Check sheet for the modelled part. Datum: model origin and axes. Units: mm. A direction names the side the tool comes from. Round coordinates to 2 decimals unless told otherwise and drop trailing zeros. Write each loop counter-clockwise with the first axis right and the second up, starting at its lowest first coordinate (ties: lowest second). Pieces come first, ordered by that corner, then holes.
Item 1: Section check B-B, the plane y = 2. State how many separate pieces and enclosed holes the cut face has, plus the area to 3 significant figures.
Item 2: Set-up check for faces 4 (the flat face through (14.75, -2, 34)), 5 (the flat face through (-10.485, -2, 0)), 6 (the flat face through (12.185, 3.2, 0.1)): record each of +Z, -Z, +X, -X, +Y, -Y from which the full face is reachable in a straight line by a thin tool's end or side.
Item 3: Material ranges on line 1 along Y through (x, z) = (0, -20); line 2 along X through (y, z) = (0.25, -7); line 3 along Y through (x, z) = (0, 35.5), recorded low to high.
Item 4: Section check C-C, the plane z = 35.5. Record the cut outline in (x, y), plus the area to 3 significant figures.
Item 5: Section check A-A, the plane z = -3. Record the cut outline in (x, y) (3 decimals).
Item 6: Depth check by flat-ended pin: pin 1 (5 mm diameter, centred on y = -1, z = -34, fed in from -X); pin 2 (1 mm diameter, centred on y = -0.5, z = -12.5, fed in from +X); pin 3 (3.5 mm diameter, centred on y = -2.5, z = -35, fed in from +X). Enter the tip coordinate at first touch or a pass-through.
Item 7: Release check for a two-part mould opening along Y. For faces 1 (the flat face through (9.7, -3, 49.2)), 2 (the flat face through (11, 0, 0)), 3 (the cylindrical face through (0, 1, 20)) record: pulls with the +Y half, pulls with the -Y half, needs draft (parallel to the pull), parting line crosses it, or undercut.
Autodesk Inventor part; units mm, degrees
ref_plane "YZ Plane" through (0, 0, 0) normal (1, 0, 0) x (0, 1, 0)
ref_plane "XZ Plane" through (0, 0, 0) normal (0, 1, 0) x (-1, 0, 0)
ref_plane "XY Plane" through (0, 0, 0) normal (0, 0, 1) x (1, 0, 0)
sketch "Chamber_outline" plane through (0, 0, 0) normal (0, 1, 0) x (-1, 0, 0)
  line L0 (0, -6.495) -> (0, 6.495) construction
  line L1 (12.185, -6.495) -> (12.185, 6.495)
  line L2 (-12.185, 6.495) -> (-12.185, -6.495)
  arc A0 (-12.185, -6.495) -> (12.185, -6.495) centre (0, -6.495) ccw
  arc A1 (12.185, 6.495) -> (-12.185, 6.495) centre (0, 6.495) ccw
  line L3 (15.7049, -6.495) -> (15.7049, 6.495)
  arc A2 (15.7049, 6.495) -> (-15.7049, 6.495) centre (0, 6.495) ccw
  line L4 (-15.7049, 6.495) -> (-15.7049, -6.495)
  arc A3 (-15.7049, -6.495) -> (15.7049, -6.495) centre (0, -6.495) ccw
  line L5 (12.185, 0) -> (-12.185, 0)
  line L6 (14.7497, -11.8886) -> (14.7497, -56.8886)
  line L7 (14.7497, -56.8886) -> (-14.7497, -56.8886)
  line L8 (-14.7497, -56.8886) -> (-14.7497, -11.8886)
  line L9 (14.7497, 11.8886) -> (14.7497, 56.8886)
  line L10 (14.7497, 56.8886) -> (-14.7497, 56.8886)
  line L11 (-14.7497, 56.8886) -> (-14.7497, 11.8886)
  line L12 (10.485, -6.495) -> (10.485, 6.495)
  arc A4 (10.485, 6.495) -> (-10.485, 6.495) centre (0, 6.495) ccw
  line L13 (-10.485, 6.495) -> (-10.485, -6.495)
  arc A5 (-10.485, -6.495) -> (10.485, -6.495) centre (0, -6.495) ccw
  point P0 (0, 0)
  point P1 (0, 0)
  point P2 (0, 0)
  point P3 (0, -56.8886)
  point P4 (0, 56.8886)
  point P5 (-14.7497, 11.8886)
  point P6 (14.7497, 11.8886)
  point P7 (0, -18.68)
  point P8 (0, 18.68)
  dimension "d18" = 24.37
  dimension "d26" = 1.7
  dimension "d58" = 45
  dimension "d82" = 37.36
extrude "Extrusion3" add sketch "Chamber_outline" along normal blind 4.5 contours A3 L4 A2 L3
extrude "Extrusion4" add sketch "Chamber_outline" along normal blind 0.5 contours L6 L7 L8 A3 | A2 L11 L10 L9
extrude "Extrusion5" add sketch "Chamber_outline" against normal blind 4 contours A0 L2 L5 L13 A5 L12 L1 | L5 L12 A4 L13 L2 A1 L1 | A3 L4 A2 L3 | L6 L7 L8 A3 | A2 L11 L10 L9
fillet "Fillet1" radius 10 2 edges at (-14.7497, -2, 11.8886) (-14.7497, 0.25, 11.8886)
fillet "Fillet2" radius 10 6 edges at (-14.7497, -2, -11.8886) (-14.7497, 0.25, -11.8886) (14.7497, 0.25, -11.8886) (14.7497, -2, -11.8886) (14.7497, 0.25, 11.8886) (14.7497, -2, 11.8886)
fillet "Fillet3" radius 2 8 edges at (-14.7497, -2, -56.8886) (-14.7497, 0.25, -56.8886) (-14.7497, -2, 56.8886) (-14.7497, 0.25, 56.8886) (14.7497, -2, 56.8886) (14.7497, 0.25, 56.8886) (14.7497, -2, -56.8886) (14.7497, 0.25, -56.8886)
sketch "Sketch9" plane through (0, -4, 0) normal (0, -1, 0) x (1, 0, 0)
  line L0 (0.801, 42.3276) -> (0.801, 45.3727) construction
  line L1 (0.801, 45.3727) -> (3.851, 45.3727) construction
  line L2 (3.851, 45.3727) -> (3.851, 42.3276) construction
  line L3 (3.851, 42.3276) -> (0.801, 42.3276) construction
  line L4 (10.801, 43.349) -> (0.801, 43.349)
  line L5 (0.801, 43.349) -> (0.801, 47.602)
  spline S0 degree 2 poles (0.801, 47.602) (0.801, 49.2102) (1.3422, 50.6584) (2.7141, 51.5349) (3.6059, 51.5349) knots 0 0 0 1 2 3 3 3
  spline S1 degree 2 poles (3.6059, 51.5349) (4.7263, 51.5349) (6.1973, 50.2163) (6.3879, 48.8977) knots 0 0 0 1 2 2 2
  spline S2 degree 2 poles (6.3879, 48.8977) (6.769, 49.5532) (7.6836, 50.4069) (8.8498, 51.131) knots 0 0 0 1 2 2 2
  line L6 (8.8498, 51.131) -> (10.801, 52.3505)
  line L7 (10.801, 52.3505) -> (10.801, 49.9343)
  line L8 (10.801, 49.9343) -> (8.6211, 48.4785)
  spline S3 degree 2 poles (8.6211, 48.4785) (7.455, 47.6935) (6.8452, 47.1218) (6.6242, 46.4816) (6.6242, 45.7804) knots 0 0 0 1 2 3 3 3
  line L9 (6.6242, 45.7804) -> (6.6242, 45.3688)
  line L10 (6.6242, 45.3688) -> (10.801, 45.3688)
  line L11 (10.801, 45.3688) -> (10.801, 43.349)
  line L12 (5.0312, 45.3688) -> (5.0312, 46.8627)
  spline S4 degree 2 poles (5.0312, 46.8627) (5.0312, 48.3185) (4.7873, 49.0426) (4.1851, 49.4541) (3.7355, 49.4541) knots 0 0 0 1 2 3 3 3
  spline S5 degree 2 poles (3.7355, 49.4541) (3.2324, 49.4541) (2.6074, 48.913) (2.5236, 48.4252) knots 0 0 0 1 2 2 2
  spline S6 degree 2 poles (2.5236, 48.4252) (2.4931, 48.1737) (2.4931, 46.9465) knots 0 0 0 1 1 1
  line L13 (2.4931, 46.9465) -> (2.4931, 45.3688)
  line L14 (2.4931, 45.3688) -> (5.0312, 45.3688)
  point P0 (0, 0)
extrude "Extrusion14" cut sketch "Sketch9" against normal blind 2
sketch "Sketch3" plane through (15.7049, 4.5, 6.495) normal (1, 0, 0) x (0, 0, -1)
  circle A0 centre (6.5, -2.5) radius 1
  line L0 (0, 0) -> (12.99, 0)
  circle A1 centre (14.5, -2.5) radius 1
  circle A2 centre (-1.5, -2.5) radius 1
  point P0 (6.495, -4.5)
  dimension "d41" = 2
  dimension "d43" = 2.5
  dimension "d85" = 2
  dimension "d86" = 2
  dimension "d87" = 8
  dimension "d88" = 8
extrude "Extrusion6" cut sketch "Sketch3" against normal through all
sketch "Sketch4" plane through (-12.7497, 0.5, 56.8886) normal (0, 0, 1) x (1, 0, 0)
  circle A0 centre (12.7497, 1.5) radius 1
  line L0 (28.4546, 4) -> (-2.9552, 4)
  point P0 (12.7497, -0.5)
  point P1 (12.7497, 4)
  dimension "d36" = 2
  dimension "d42" = 2.5
extrude "Extrusion7" cut sketch "Sketch4" against normal through all
sketch "Sketch5" plane through (0, -4, 0) normal (0, -1, 0) x (1, 0, 0)
  line L0 (-10.485, -6.495) -> (-10.485, 6.495)
  line L1 (-10.485, -6.495) -> (-8.4271, -6.495)
  line L2 (-7.9121, 0.245) -> (-7.9121, 6.495)
  line L3 (-7.9121, 6.495) -> (-10.485, 6.495)
  line L4 (10.485, -6.495) -> (10.485, 6.495)
  line L5 (10.485, -6.495) -> (8.4271, -6.495)
  line L6 (8.3305, -0.2609) -> (8.3305, 6.495)
  line L7 (8.3305, 6.495) -> (10.485, 6.495)
  arc A0 (10.485, 6.495) -> (-10.485, 6.495) centre (0, 6.495) ccw
  arc A1 (-10.485, -6.495) -> (10.485, -6.495) centre (0, -6.495) ccw
  arc A2 (-10.485, -6.495) -> (10.485, -6.495) centre (0, -6.495) ccw
  line L8 (-7.079, -14.2295) -> (-5.3711, -11.1831)
  line L9 (-5.3711, -11.1831) -> (-3.3516, -12.3154)
  line L10 (-3.3516, -12.3154) -> (-5.1945, -15.6028)
  line L11 (-7.4267, 14.3644) -> (-5.7188, 11.3181)
  line L12 (-5.7188, 11.3181) -> (-3.6001, 12.5059)
  line L13 (-3.6001, 12.5059) -> (-5.4497, 15.8051)
  line L14 (3.586, 12.9764) -> (5.1976, 15.6011)
  line L15 (5.8011, 11.7346) -> (3.586, 12.9764)
  line L16 (7.1611, 14.1536) -> (5.8011, 11.7346)
  line L17 (-10.485, -6.495) -> (10.8395, -6.495)
  line L18 (1.9666, 16.7939) -> (1.9666, -0.2609)
  line L19 (-2.0003, -16.7874) -> (-2.0003, -6.495)
  line L20 (-1.0812, 0.245) -> (-1.0812, 16.9241)
  line L21 (4.8643, -15.7834) -> (4.8643, -6.495)
  line L22 (-7.9121, 0.245) -> (-1.0812, 0.245)
  line L23 (1.9666, -0.2609) -> (8.3305, -0.2609)
  point P0 (0, 0)
  point P1 (1.5355, -6.495)
  point P2 (-7.079, -14.2295)
  point P3 (-5.1945, -15.6028)
  point P4 (-5.3016, 15.5409)
  point P5 (-7.2574, 14.0624)
  point P6 (7.5128, 14.2848)
  point P7 (5.4529, 15.8033)
  point P8 (8.4271, -6.495)
  point P9 (4.8643, -15.7834)
sketch "Sketch6" plane through (0, -4, 0) normal (0, -1, 0) x (1, 0, 0)
  ellipse E0 centre (0, -5) end of major axis (0.355, -4.9802) minor radius 0.3556
  circle A0 centre (1, -5.9999) radius 0.3556
  circle A1 centre (0, -5.9999) radius 0.3556
  circle A2 centre (-1, -6) radius 0.3556
  circle A3 centre (-1, -4.9999) radius 0.3556
  circle A4 centre (1, -5) radius 0.3556
  circle A5 centre (1, -6.9999) radius 0.3556
  ellipse E1 centre (0, -7) end of major axis (0.3551, -6.9801) minor radius 0.3556
  ellipse E2 centre (-1, -7) end of major axis (-0.645, -6.9801) minor radius 0.3556
  ellipse E3 centre (6, -3) end of major axis (6.355, -2.9802) minor radius 0.3556
  circle A6 centre (5, -3) radius 0.3556
  ellipse E4 centre (4, -2.9999) end of major axis (4.3551, -2.9801) minor radius 0.3556
  circle A7 centre (4, -4) radius 0.3556
  ellipse E5 centre (5, -4) end of major axis (5.355, -3.9802) minor radius 0.3556
  ellipse E6 centre (6, -3.9999) end of major axis (6.3551, -3.9801) minor radius 0.3556
  circle A8 centre (6, -2) radius 0.3556
  circle A9 centre (5, -2) radius 0.3556
  circle A10 centre (4, -1.9999) radius 0.3556
  circle A11 centre (3, -12) radius 0.3556
  circle A12 centre (4, -11.9999) radius 0.3556
  circle A13 centre (3, -10.9999) radius 0.3556
  circle A14 centre (4, -11) radius 0.3556
  circle A15 centre (2, -10.9999) radius 0.3556
  circle A16 centre (2, -12) radius 0.3556
  circle A17 centre (2, -13) radius 0.3555
  ellipse E7 centre (3, -13) end of major axis (3.0198, -13.355) minor radius 0.3556
  ellipse E8 centre (4, -13) end of major axis (4.0198, -13.355) minor radius 0.3556
  circle A18 centre (1.5, 9) radius 0.3556
  circle A19 centre (1.5, 8) radius 0.3556
  circle A20 centre (0.5, 8) radius 0.3556
  ellipse E9 centre (-0.5, 8.0001) end of major axis (-0.1449, 8.0199) minor radius 0.3556
  circle A21 centre (-0.5, 9) radius 0.3556
  circle A22 centre (-0.5, 10) radius 0.3556
  circle A23 centre (1.5, 10.0001) radius 0.3556
  ellipse E10 centre (0.5, 10) end of major axis (0.5198, 9.645) minor radius 0.3556
  circle A24 centre (0.5, 9) radius 0.3556
  circle A25 centre (3, -12) radius 0.4056
  circle A26 centre (0, -5.9999) radius 0.4056
  circle A27 centre (5, -3) radius 0.4056
  circle A28 centre (0.5, 9) radius 0.4056
  circle A29 centre (-1, -6) radius 0.4056
  point P0 (0, 0)
  dimension "d63" = 0.05
  dimension "d64" = 0.05
  dimension "d65" = 0.05
  dimension "d66" = 0.05
  dimension "d77" = 0.05
sketch "Sketch7" plane through (0, -0.5, 0) normal (0, 1, 0) x (1, 0, 0)
  arc A0 (12.185, 6.495) -> (-12.185, 6.495) centre (0, 6.495) ccw
  arc A1 (10.285, 6.495) -> (-10.285, 6.495) centre (0, 6.495) ccw
  line L0 (-10.485, -6.495) -> (-10.485, 6.495)
  arc A2 (10.485, 6.495) -> (-10.485, 6.495) centre (0, 6.495) ccw
  line L1 (10.485, 6.495) -> (10.485, -6.495)
  arc A3 (-10.485, -6.495) -> (10.485, -6.495) centre (0, -6.495) ccw
  line L2 (-12.185, -6.495) -> (-12.185, 6.495)
  arc A4 (-12.185, -6.495) -> (12.185, -6.495) centre (0, -6.495) ccw
  line L3 (12.185, 6.495) -> (12.185, -6.495)
  arc A5 (12.185, 6.495) -> (-12.185, 6.495) centre (0, 6.495) ccw
  arc A6 (-12.185, -6.495) -> (12.185, -6.495) centre (0, -6.495) ccw
  line L4 (12.185, 6.495) -> (12.185, -6.495)
  line L5 (-12.185, -6.495) -> (-12.185, 6.495)
  line L6 (-10.285, -6.495) -> (-10.285, 6.495)
  arc A7 (10.285, 6.495) -> (-10.285, 6.495) centre (0, 6.495) ccw
  line L7 (10.285, 6.495) -> (10.285, -6.495)
  arc A8 (-10.285, -6.495) -> (10.285, -6.495) centre (0, -6.495) ccw
  circle A9 centre (5, 3) radius 0.4056
  circle A10 centre (0, 5.9999) radius 0.4056
  circle A11 centre (0.5, -9) radius 0.4056
  circle A12 centre (3, 12) radius 0.4056
  line L8 (10.485, 6.495) -> (4.8643, 6.495)
  line L9 (4.8643, 6.495) -> (4.8643, 15.7834)
  arc A13 (4.8643, 15.7834) -> (-2.0003, 16.7874) centre (0, 6.495) ccw
  line L10 (-2.0003, 16.7874) -> (-2.0003, 6.495)
  line L11 (-2.0003, 6.495) -> (-10.485, 6.495)
  line L12 (-10.485, -6.495) -> (-10.485, 6.495)
  line L13 (-10.485, -6.495) -> (-7.9121, -6.495)
  line L14 (-7.9121, -6.495) -> (-7.9121, -0.245)
  line L15 (-7.9121, -0.245) -> (-1.0812, -0.245)
  line L16 (-1.0812, -0.245) -> (-1.0812, -16.9241)
  arc A14 (-1.0812, -16.9241) -> (1.9666, -16.7939) centre (0, -6.495) ccw
  line L17 (1.9666, -16.7939) -> (1.9666, 0.2609)
  line L18 (1.9666, 0.2609) -> (8.3305, 0.2609)
  line L19 (8.3305, 0.2609) -> (8.3305, -6.495)
  line L20 (8.3305, -6.495) -> (10.485, -6.495)
  line L21 (10.485, 6.495) -> (10.485, -6.495)
  line L22 (7.1611, -14.1536) -> (5.8011, -11.7346)
  line L23 (5.8011, -11.7346) -> (3.586, -12.9764)
  line L24 (3.586, -12.9764) -> (5.1976, -15.6011)
  arc A15 (5.1976, -15.6011) -> (7.1611, -14.1536) centre (0, -6.495) ccw
  line L25 (-7.079, 14.2295) -> (-5.3711, 11.1831)
  line L26 (-5.3711, 11.1831) -> (-3.3516, 12.3154)
  line L27 (-3.3516, 12.3154) -> (-5.1945, 15.6028)
  arc A16 (-5.1945, 15.6028) -> (-7.079, 14.2295) centre (0, 6.495) ccw
  line L28 (-5.3016, -15.5409) -> (-3.6001, -12.5059)
  line L29 (-3.6001, -12.5059) -> (-5.7188, -11.3181)
  line L30 (-5.7188, -11.3181) -> (-7.2574, -14.0624)
  arc A17 (-7.2574, -14.0624) -> (-5.3016, -15.5409) centre (0, -6.495) ccw
  circle A18 centre (-1, 6) radius 0.4056
  line L31 (0, -16.78) -> (0, 0)
  line L32 (-10.285, 0) -> (0, 0)
  line L33 (0, 0) -> (10.285, 0)
  line L34 (0, 0) -> (0, 16.78)
  point P0 (-1.0812, -16.723)
  point P1 (1.9666, -16.5902)
  point P2 (10.285, -6.495)
  point P3 (10.285, 6.495)
  point P4 (4.8643, 15.557)
  point P5 (-2.0003, 16.5836)
  point P6 (-10.285, 6.495)
  point P7 (-10.285, -6.495)
  point P8 (5.0929, -15.4305)
  point P9 (7.0601, -13.974)
  point P10 (-7.1563, -13.8821)
  point P11 (-5.2037, -15.3664)
  point P12 (-5.0967, 15.4283)
  point P13 (-6.9785, 14.0503)
  dimension "d83" = 33.56
equation "\"metal_holder_thickness\" = 5"
equation "\"metal_holder_slot_length\" = 5"
properties part number "holder_base"
Values found:
1. separate pieces: 8
1. enclosed holes: 0
1. area: 343 mm2
2. face 4: +Z, +X, +Y, -Y
2. face 5: +Y, -Y
2. face 6: +Y
3. line 1: y = -4 to 1, 3 to 4.5
3. line 2: x = -15.7 to -12.17, 12.17 to 15.7
3. line 3: y = -4 to 0.5
4. outline: (-14.75, -4) - (14.75, -4) - (14.75, 0.5) - (-14.75, 0.5) - close
4. area: 133 mm2
5. outline: (-15.705, -4) - (-10.485, -4) - (-10.485, 0) - (-12.185, 0) - (-12.185, 4.5) - (-15.705, 4.5) - close; (10.485, -4) - (15.705, -4) - (15.705, 4.5) - (12.185, 4.5) - (12.185, 0) - (10.485, 0) - close
6. pin 1: stops at x = -14.75
6. pin 2: stops at x = 14.85
6. pin 3: stops at x = 14.75
7. face 1: needs draft
7. face 2: pulls with the +Y half
7. face 3: undercut
